Build history of the part. All positions in model axes, mm. Give positions to 0.01 mm unless a question says otherwise; leave off trailing zeros. Loops run counter-clockwise (first coordinate to the right, second up) from the corner with the lowest first, then second, coordinate; pieces in that order, holes last. Notation, with made-up numbers: (-21.5, 25) -> (-1.5, 25) arc R18 cw to (-1.5, 59) -> close; hole circle Ø7 at (45, 12.25). An arc over 180 degrees is marked (long way). Answer as a JSON object with one key per item and string values. Group by question number.
Q1. Drop flat-ended pins along their axis: pin 1 (1 mm diameter, centred on x = 123, z = 1, fed in from -Y); pin 2 (1.6 mm diameter, centred on x = 123, z = 1.5, fed in from +Y); pin 3 (1 mm diameter, centred on y = 1.5, z = 1, fed in from -X). Give the stop position or say it passes through.
Q2. Band-saw the part on C-C, the plane x = 30.5. Write the cut outline in (y, z) (3 decimals), plus the area to 3 significant figures.
Q3. Band-saw the part on B-B, the plane z = 0.5. Count the separate pieces of the cut face and the enclosed holes in it, plus the area to 3 significant figures.
Q4. Band-saw the part on A-A, the plane x = 74.5. Write the cut outline in (y, z) (3 decimals).
Q5. Wall check: probe 1 along Y at (x, z) = (21.5, 2.7) (3 decimals); probe 2 along Y at (x, z) = (296, 0.25). Give the ranges that are in metal, low to high. Write a range as from..to.
from build123d import *

# Parameters (mm, degrees)
SKETCH1_W           = 12.9
SKETCH1_H           = 3.3782
BOSS_EXTRUDE1_DEPTH = 3.175


with BuildPart() as part:
    # Sketch1 → Boss-Extrude1 (new body)
    with BuildSketch(Plane.XY):
        Polygon((3.0496002, 100.7618), (0, 100.7618), (0, -6.3246), (3.0496002, -6.3246), (3.0496002, -3.2782), (406.4, -3.2782), (406.4, 97.7154), (3.0496002, 97.7154), align=None)
        with Locations((19.05, 92.8513)):
            Rectangle(SKETCH1_W, SKETCH1_H, mode=Mode.SUBTRACT)
        with Locations((45.357142857, 92.8513)):
            Rectangle(SKETCH1_W, SKETCH1_H, mode=Mode.SUBTRACT)
        with Locations((387.35, 92.8513)):
            Rectangle(SKETCH1_W, SKETCH1_H, mode=Mode.SUBTRACT)
        with Locations((361.042857143, 92.8513)):
            Rectangle(SKETCH1_W, SKETCH1_H, mode=Mode.SUBTRACT)
        with Locations((71.664285714, 92.8513)):
            Rectangle(SKETCH1_W, SKETCH1_H, mode=Mode.SUBTRACT)
        with Locations((97.971428571, 92.8513)):
            Rectangle(SKETCH1_W, SKETCH1_H, mode=Mode.SUBTRACT)
        with Locations((124.278571429, 92.8513)):
            Rectangle(SKETCH1_W, SKETCH1_H, mode=Mode.SUBTRACT)
        with Locations((150.585714286, 92.8513)):
            Rectangle(SKETCH1_W, SKETCH1_H, mode=Mode.SUBTRACT)
        with Locations((176.892857143, 92.8513)):
            Rectangle(SKETCH1_W, SKETCH1_H, mode=Mode.SUBTRACT)
        with Locations((203.2, 92.8513)):
            Rectangle(SKETCH1_W, SKETCH1_H, mode=Mode.SUBTRACT)
        with Locations((229.507142857, 92.8513)):
            Rectangle(SKETCH1_W, SKETCH1_H, mode=Mode.SUBTRACT)
        with Locations((255.814285714, 92.8513)):
            Rectangle(SKETCH1_W, SKETCH1_H, mode=Mode.SUBTRACT)
        with Locations((282.121428571, 92.8513)):
            Rectangle(SKETCH1_W, SKETCH1_H, mode=Mode.SUBTRACT)
        with Locations((308.428571429, 92.8513)):
            Rectangle(SKETCH1_W, SKETCH1_H, mode=Mode.SUBTRACT)
        with Locations((334.735714286, 92.8513)):
            Rectangle(SKETCH1_W, SKETCH1_H, mode=Mode.SUBTRACT)
        with Locations((387.35, 1.5859)):
            Rectangle(SKETCH1_W, SKETCH1_H, mode=Mode.SUBTRACT)
        with Locations((361.042857143, 1.5859)):
            Rectangle(SKETCH1_W, SKETCH1_H, mode=Mode.SUBTRACT)
        with Locations((334.735714286, 1.5859)):
            Rectangle(SKETCH1_W, SKETCH1_H, mode=Mode.SUBTRACT)
        with Locations((308.428571429, 1.5859)):
            Rectangle(SKETCH1_W, SKETCH1_H, mode=Mode.SUBTRACT)
        with Locations((282.121428571, 1.5859)):
            Rectangle(SKETCH1_W, SKETCH1_H, mode=Mode.SUBTRACT)
        with Locations((255.814285714, 1.5859)):
            Rectangle(SKETCH1_W, SKETCH1_H, mode=Mode.SUBTRACT)
        with Locations((229.507142857, 1.5859)):
            Rectangle(SKETCH1_W, SKETCH1_H, mode=Mode.SUBTRACT)
        with Locations((203.2, 1.5859)):
            Rectangle(SKETCH1_W, SKETCH1_H, mode=Mode.SUBTRACT)
        with Locations((176.892857143, 1.5859)):
            Rectangle(SKETCH1_W, SKETCH1_H, mode=Mode.SUBTRACT)
        with Locations((150.585714286, 1.5859)):
            Rectangle(SKETCH1_W, SKETCH1_H, mode=Mode.SUBTRACT)
        with Locations((124.278571429, 1.5859)):
            Rectangle(SKETCH1_W, SKETCH1_H, mode=Mode.SUBTRACT)
        with Locations((97.971428571, 1.5859)):
            Rectangle(SKETCH1_W, SKETCH1_H, mode=Mode.SUBTRACT)
        with Locations((71.664285714, 1.5859)):
            Rectangle(SKETCH1_W, SKETCH1_H, mode=Mode.SUBTRACT)
        with Locations((45.357142857, 1.5859)):
            Rectangle(SKETCH1_W, SKETCH1_H, mode=Mode.SUBTRACT)
        with Locations((19.05, 1.5859)):
            Rectangle(SKETCH1_W, SKETCH1_H, mode=Mode.SUBTRACT)
    extrude(amount=BOSS_EXTRUDE1_DEPTH)


solid = part.part
Worked answers:
{
 "1": {"pin 1": "y = -3.28", "pin 2": "y = 97.72", "pin 3": "x = 0"},
 "2": {"outline": "(-3.278, 0) -> (97.715, 0) -> (97.715, 3.175) -> (-3.278, 3.175) -> close", "area": "321 mm2"},
 "3": {"separate pieces": "1", "enclosed holes": "30", "area": "39,800 mm2"},
 "4": {"outline": "(-3.278, 0) -> (-0.103, 0) -> (-0.103, 3.175) -> (-3.278, 3.175) -> close; (3.275, 0) -> (91.162, 0) -> (91.162, 3.175) -> (3.275, 3.175) -> close; (94.54, 0) -> (97.715, 0) -> (97.715, 3.175) -> (94.54, 3.175) -> close"},
 "5": {"probe 1": "-3.278..-0.103, 3.275..91.162, 94.54..97.715", "probe 2": "-3.28..97.72"}
}
